```python
from build123d import *

# Parameters (mm, degrees)
CROQUIS1_W              = 12.5
CROQUIS1_H              = 25
CROQUIS1_W_2            = 25
SALIENTE_EXTRUIR1_DEPTH = 10
CROQUIS1_3_W            = 25
CROQUIS1_3_H            = 25
SALIENTE_EXTRUIR2_DEPTH = 105
CROQUIS2_R              = 4.15
CORTAR_EXTRUIR1_DEPTH   = 60
CROQUIS3_R              = 2.1
CORTAR_EXTRUIR2_DEPTH   = 10
CROQUIS1_4_W            = 50
CROQUIS1_4_H            = 12.5
SALIENTE_EXTRUIR3_DEPTH = 10
CROQUIS5_R              = 1.5
CORTAR_EXTRUIR4_DEPTH   = 10
CORTAR_EXTRUIR7_DEPTH   = 10
CROQUIS8_R              = 2.1
CORTAR_EXTRUIR9_DEPTH   = 15
CROQUIS9_R              = 1.5
CORTAR_EXTRUIR10_DEPTH  = 10
SALIENTE_EXTRUIR4_DEPTH = 12.5


with BuildPart() as part:
    # Croquis1 → Saliente-Extruir1 (new body)
    with BuildSketch(Plane(origin=(0, 0, 0), x_dir=(1, 0, 0), z_dir=(0, 1, 0))):
        with Locations((-18.75, 0)):
            Rectangle(CROQUIS1_W, CROQUIS1_H)
        with Locations((18.75, 0)):
            Rectangle(CROQUIS1_W, CROQUIS1_H)
        Rectangle(CROQUIS1_W_2, CROQUIS1_H)
    extrude(amount=SALIENTE_EXTRUIR1_DEPTH)

    # Croquis1_3 → Saliente-Extruir2 (add)
    with BuildSketch(Plane(origin=(0, 0, 0), x_dir=(1, 0, 0), z_dir=(0, 1, 0))):
        Rectangle(CROQUIS1_3_W, CROQUIS1_3_H)
    extrude(amount=SALIENTE_EXTRUIR2_DEPTH)

    # Croquis2 → Cortar-Extruir1 (cut)
    with BuildSketch(Plane.XY.offset(12.5)):
        with Locations((0, 90)):
            Circle(CROQUIS2_R)
    extrude(amount=-CORTAR_EXTRUIR1_DEPTH, mode=Mode.SUBTRACT)

    # Croquis3 → Cortar-Extruir2 (cut)
    with BuildSketch(Plane(origin=(12.5, 0, 0), x_dir=(0, 0, -1), z_dir=(1, 0, 0))):
        with Locations((0, 90)):
            Circle(CROQUIS3_R)
    extrude(amount=-CORTAR_EXTRUIR2_DEPTH, mode=Mode.SUBTRACT)

    # Croquis1_4 → Saliente-Extruir3 (add)
    with BuildSketch(Plane(origin=(0, 0, 0), x_dir=(1, 0, 0), z_dir=(0, 1, 0))):
        with Locations((0, 18.75)):
            Rectangle(CROQUIS1_4_W, CROQUIS1_4_H)
        with Locations((0, -18.75)):
            Rectangle(CROQUIS1_4_W, CROQUIS1_4_H)
    extrude(amount=SALIENTE_EXTRUIR3_DEPTH)

    # Croquis5 → Cortar-Extruir4 (cut)
    with BuildSketch(Plane(origin=(0, 10, 0), x_dir=(1, 0, 0), z_dir=(0, 1, 0))):
        with Locations((-4.456486884, 18.75)):
            Circle(CROQUIS5_R)
        with Locations((-4.456486884, -18.75)):
            Circle(CROQUIS5_R)
    extrude(amount=-CORTAR_EXTRUIR4_DEPTH, mode=Mode.SUBTRACT)

    # Croquis6 → Cortar-Extruir7 (cut)
    with BuildSketch(Plane(origin=(0, 10, 0), x_dir=(1, 0, 0), z_dir=(0, 1, 0))):
        Polygon((-12.5, 25), (-12.5, 12.5), (-12.5, -12.5), (-12.5, -25), (-25, -25), (-25, 25), align=None)
    extrude(amount=-CORTAR_EXTRUIR7_DEPTH, mode=Mode.SUBTRACT)

    # Croquis8 → Cortar-Extruir9 (cut)
    with BuildSketch(Plane(origin=(0, 105, 0), x_dir=(1, 0, 0), z_dir=(0, 1, 0))):
        Circle(CROQUIS8_R)
    extrude(amount=-CORTAR_EXTRUIR9_DEPTH, mode=Mode.SUBTRACT)

    # Croquis9 → Cortar-Extruir10 (cut)
    with BuildSketch(Plane(origin=(0, 10, 0), x_dir=(1, 0, 0), z_dir=(0, 1, 0))):
        with Locations((19, -18.75)):
            Circle(CROQUIS9_R)
        with Locations((19, 18.75)):
            Circle(CROQUIS9_R)
    extrude(amount=-CORTAR_EXTRUIR10_DEPTH, mode=Mode.SUBTRACT)

    # Croquis10 → Saliente-Extruir4 (add, symmetric)
    with BuildSketch(Plane.XY):
        Polygon((12.5, 10), (25, 10), (12.5, 70), align=None)
    extrude(amount=SALIENTE_EXTRUIR4_DEPTH, both=True)


solid = part.part
```
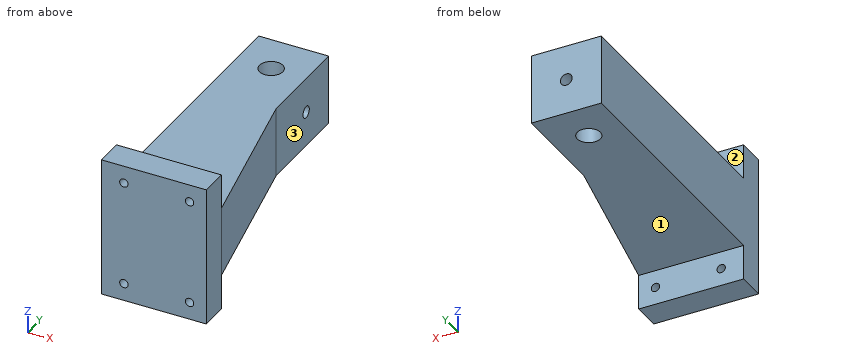
Geometry: final body of the model. Coordinates: model frame, mm. Face numbers are marked on the shaded views. A direction names the side the tool comes from. Give positions to 0.01 mm unless a question says otherwise; leave off trailing zeros. Write each loop counter-clockwise with the first axis right and the second up, starting at its lowest first coordinate (ties: lowest second). Pieces come first, ordered by that corner, then holes.
1. Reachability of the marked faces 1, 2 and 3 from +Z, -Z, +X, -X, +Y, -Y: full face, straight path, thin tool, end or side. Return the list, or none.
2. Pin query (flat end, axial travel): P1, Ø6, axis at x = 12, z = 18.5, coming from the +Y side; P2, Ø2, axis at x = 5.5, y = 19, coming from the -Z side; P3, Ø20, axis at y = 87, z = 3.5, coming from the +X side. Return the tip coordinate at first contact, or that it passes through.
3. Section query A-A, the plane z = -18.75. Return loops of the section in (x, y).
4. Section query C-C, the plane z = 0. Return loops of the section in (x, y), then the cut area to 3 significant figures.
5. Section query D-D, the plane x = 9.5. Return loops of the section in (y, z), then the cut area to 3 significant figures.
6. Section query B-B, the plane x = 0. Return loops of the section in (y, z), then the cut area to 3 significant figures.
7. Line query: probe 1 along Z at (x, y) = (19, 3.75); probe 2 along X at (y, z) = (6.25, 18.75); probe 3 along X at (y, z) = (101.5, 0). Output: solid intervals per line, ascending.
Computed:
1. face 1: -Z, +X, -X, +Y
1. face 2: +Z, +X, -X, +Y
1. face 3: +Z, -Z, +X, +Y
2. P1: stops at y = 10
2. P2: stops at z = -12.5
2. P3: stops at x = 12.5
3. outline: (-12.5, 0) - (-5.96, 0) - (-5.96, 10) - (-12.5, 10) - close; (-2.96, 0) - (17.5, 0) - (17.5, 10) - (-2.96, 10) - close; (20.5, 0) - (25, 0) - (25, 10) - (20.5, 10) - close
4. outline: (-12.5, 0) - (25, 0) - (25, 10) - (12.5, 70) - (12.5, 87.9) - (3.58, 87.9) arc R4.15 cw (long way) to (-2.1, 93.58) - (-2.1, 105) - (-12.5, 105) - close; (2.1, 93.58) arc R4.15 cw to (3.58, 92.1) - (12.5, 92.1) - (12.5, 105) - (2.1, 105) - close
4. area: 2,990 mm2
5. outline: (0, -25) - (10, -25) - (10, -12.5) - (105, -12.5) - (105, 12.5) - (10, 12.5) - (10, 25) - (0, 25) - close; hole circle Ø4.2 at (90, 0)
5. area: 2,860 mm2
6. outline: (0, -25) - (10, -25) - (10, -12.5) - (85.85, -12.5) - (85.85, 12.5) - (10, 12.5) - (10, 25) - (0, 25) - close; (94.15, -12.5) - (105, -12.5) - (105, -2.1) - (94.15, -2.1) - close; (94.15, 2.1) - (105, 2.1) - (105, 12.5) - (94.15, 12.5) - close
6. area: 2,620 mm2
7. probe 1: z = -25 to -20.25, -17.25 to 17.25, 20.25 to 25
7. probe 2: x = -12.5 to -5.96, -2.96 to 17.5, 20.5 to 25
7. probe 3: x = -12.5 to -2.1, 2.1 to 12.5
